from build123d import *

# Parameters (mm, degrees)
SKETCH1_W           = 45
SKETCH1_H           = 45
SKETCH1_R           = 2.6
BOSS_EXTRUDE1_DEPTH = 7.5
SKETCH2_R           = 8.1
CUT_EXTRUDE1_DEPTH  = 6
CUT_EXTRUDE4_START  = -6
SKETCH5_R           = 8.1
CUT_EXTRUDE4_DEPTH  = 6
SKETCH7_W           = 37
SKETCH7_H           = 7
BOSS_EXTRUDE2_DEPTH = 10
CUT_EXTRUDE6_START  = 2
CUT_EXTRUDE6_DEPTH  = 3.6
CUT_EXTRUDE7_START  = -2
SKETCH8_R           = 2.1
CUT_EXTRUDE7_DEPTH  = 41.278836313
SKETCH9_W           = 3
SKETCH9_H           = 7
BOSS_EXTRUDE3_DEPTH = 10
SKETCH10_W          = 7
SKETCH10_H          = 7
BOSS_EXTRUDE4_DEPTH = 2
CHAMFER2_SIZE2      = 7
CHAMFER2_SIZE       = 2
CHAMFER3_SIZE2      = 7
CHAMFER3_SIZE       = 2


with BuildPart() as part:
    # Sketch1 → Boss-Extrude1 (new, symmetric)
    with BuildSketch(Plane.XY):
        Rectangle(SKETCH1_W, SKETCH1_H)
        Circle(SKETCH1_R, mode=Mode.SUBTRACT)
    extrude(amount=BOSS_EXTRUDE1_DEPTH, both=True)

    # Sketch2 → Cut-Extrude1 (cut)
    with BuildSketch(Plane.XY.offset(7.5)):
        Circle(SKETCH2_R)
    extrude(amount=-CUT_EXTRUDE1_DEPTH, mode=Mode.SUBTRACT)

    # Sketch5 → Cut-Extrude4 (cut)
    with BuildSketch(Plane(origin=(0, 0, -7.5), x_dir=(-1, 0, 0), z_dir=(0, 0, -1)).offset(CUT_EXTRUDE4_START)):
        with Locations(Location((0, 0, 0), (0, 0, 180))):
            Circle(SKETCH5_R)
    extrude(amount=CUT_EXTRUDE4_DEPTH, mode=Mode.SUBTRACT)

    # Sketch7 → Boss-Extrude2 (add)
    with BuildSketch(Plane.XZ.offset(22.5)):
        Rectangle(SKETCH7_W, SKETCH7_H)
    extrude(amount=BOSS_EXTRUDE2_DEPTH)

    # Sketch6 → Cut-Extrude6 (cut)
    with BuildSketch(Plane.XY.offset(-7.5).offset(CUT_EXTRUDE6_START)):
        Polygon((19.2, 17.636195996), (15.5, 19.772391992), (11.8, 17.636195996), (11.8, 13.363804004), (15.5, 11.227608008), (19.2, 13.363804004), align=None)
        Polygon((-11.8, 17.636195996), (-15.5, 19.772391992), (-19.2, 17.636195996), (-19.2, 13.363804004), (-15.5, 11.227608008), (-11.8, 13.363804004), align=None)
        Polygon((19.2, -13.363804004), (15.5, -11.227608008), (11.8, -13.363804004), (11.8, -17.636195996), (15.5, -19.772391992), (19.2, -17.636195996), align=None)
        Polygon((-11.8, -13.363804004), (-15.5, -11.227608008), (-19.2, -13.363804004), (-19.2, -17.636195996), (-15.5, -19.772391992), (-11.8, -17.636195996), align=None)
    extrude(amount=CUT_EXTRUDE6_DEPTH, mode=Mode.SUBTRACT)

    # Sketch8 → Cut-Extrude7 (cut, through all)
    with BuildSketch(Plane(origin=(0, 0, -7.5), x_dir=(-1, 0, 0), z_dir=(0, 0, -1)).offset(CUT_EXTRUDE7_START)):
        with Locations((-15.5, 15.5)):
            Circle(SKETCH8_R)
        with Locations((15.5, 15.5)):
            Circle(SKETCH8_R)
        with Locations((15.5, -15.5)):
            Circle(SKETCH8_R)
        with Locations((-15.5, -15.5)):
            Circle(SKETCH8_R)
    extrude(amount=-CUT_EXTRUDE7_DEPTH, mode=Mode.SUBTRACT)

    # Sketch9 → Boss-Extrude3 (add)
    with BuildSketch(Plane.XZ.offset(32.5)):
        with Locations((-17, 0)):
            Rectangle(SKETCH9_W, SKETCH9_H)
        with Locations((17, 0)):
            Rectangle(SKETCH9_W, SKETCH9_H)
    extrude(amount=BOSS_EXTRUDE3_DEPTH)

    # Sketch10 → Boss-Extrude4 (add)
    with BuildSketch(Plane.ZY.offset(18.5)):
        with Locations((0, -39)):
            Rectangle(SKETCH10_W, SKETCH10_H)
    boss_extrude4 = extrude(amount=BOSS_EXTRUDE4_DEPTH)

    # Mirror1: Boss-Extrude4 across plane
    add(boss_extrude4.mirror(Plane(origin=(0, 0, 0), x_dir=(0, 0, 1), z_dir=(1, 0, 0))))

    # Chamfer2
    chamfer2_edges = [part.edges().sort_by_distance(p)[0] for p in [
        (-20.5, -42.5, 0),
    ]]
    chamfer2_side = [part.faces().sort_by_distance(p)[0] for p in [
        (-20.46, -42.5, 0),
    ]]
    chamfer(chamfer2_edges, length=CHAMFER2_SIZE - 0.0001, length2=CHAMFER2_SIZE2 - 0.0001, reference=chamfer2_side[0])  # a hair under: the kernel refuses the full size

    # Chamfer3
    chamfer3_edges = [part.edges().sort_by_distance(p)[0] for p in [
        (20.5, -42.5, 0),
    ]]
    chamfer3_side = [part.faces().sort_by_distance(p)[0] for p in [
        (20.46, -42.5, 0),
    ]]
    chamfer(chamfer3_edges, length=CHAMFER3_SIZE - 0.0001, length2=CHAMFER3_SIZE2 - 0.0001, reference=chamfer3_side[0])  # a hair under: the kernel refuses the full size


solid = part.part
Verification items for the finished model (mm, model axes). A direction names the side the tool comes from. Round coordinates to 2 decimals unless told otherwise and drop trailing zeros. Loops run counter-clockwise (first coordinate to the right, second up) from the corner with the lowest first, then second, coordinate; pieces in that order, holes last. Notation, with made-up numbers: (25, -34) - (31, -34) arc R29 ccw to (31, -13) - close; hole circle Ø7 at (66.5, 80.25). An arc over 180 degrees is marked (long way). Answer in a Markdown table with one row per item. Add a question column.
Q1. Material ranges on line 1 (Y direction, x = 15.5, z = 4.25); line 2 (Y direction, x = 0, z = -4.75); line 3 (Z direction, x = 14, y = 12.5), recorded low to high.
Q2. Release check for a two-part mould opening along Z. For faces 5 (the face through (15.5, -37, 0)), 6 (the face through (11.8, 16, -4)), 7 (the face through (0, 10, 7.5)) record: pulls with the +Z half, pulls with the -Z half, needs draft (parallel to the pull), parting line crosses it, or undercut.
Q3. Section check B-B on x = 0. Enter the section's corners in (y, z).
Q4. Section check D-D on x = -9. Enter the section's corners in (y, z), plus the area to 3 significant figures.
Q5. Section check C-C on y = 15.5. Enter the section's corners in (x, z), plus the area to 3 significant figures.
Q6. Gauge pin test, flat ends, axial feed: pin 1 (3.5 mm diameter, centred on y = -28, z = 0, fed in from -X); pin 2 (1.5 mm diameter, centred on x = 11, z = 0, fed in from -Y); pin 3 (2 mm diameter, centred on x = 5, y = -35, fed in from +Z); pin 4 (3.5 mm diameter, centred on y = -30.5, z = -1.5, fed in from +X). Record the tip position at first contact, or that the pin passes through.
Q7. Section check A-A on z = 4.75. Enter the section's corners in (x, y).
Q8. Tool access check on faces 1 (the face through (-18.5, -29, 0)), 2 (the face through (-1.756, 7.907, -4.458)), 3 (the face through (19.2, 15, -4)), 4 (the face through (-15.5, -37, 0)). Record the directions out of +Z, -Z, +X, -X, +Y, -Y that give a thin tool (end or side, any length) a straight path to the whole face; none if there is none.
Found:
| question | item | result |
|---|---|---|
| 1 | line 1 | y = -22.5 to -17.6, -13.4 to 13.4, 17.6 to 22.5 |
| 1 | line 2 | y = -22.5 to -8.1, 8.1 to 22.5 |
| 1 | line 3 | z = -7.5 to -5.5, -1.9 to 7.5 |
| 2 | face 5 | needs draft |
| 2 | face 6 | undercut |
| 2 | face 7 | pulls with the +Z half |
| 3 | outline | (-32.5, -3.5) - (-22.5, -3.5) - (-22.5, -7.5) - (-8.1, -7.5) - (-8.1, -1.5) - (-2.6, -1.5) - (-2.6, 1.5) - (-8.1, 1.5) - (-8.1, 7.5) - (-22.5, 7.5) - (-22.5, 3.5) - (-32.5, 3.5) - close; (2.6, -1.5) - (8.1, -1.5) - (8.1, -7.5) - (22.5, -7.5) - (22.5, 7.5) - (8.1, 7.5) - (8.1, 1.5) - (2.6, 1.5) - close |
| 4 | outline | (-32.5, -3.5) - (-22.5, -3.5) - (-22.5, -7.5) - (22.5, -7.5) - (22.5, 7.5) - (-22.5, 7.5) - (-22.5, 3.5) - (-32.5, 3.5) - close |
| 4 | area | 745 mm² |
| 5 | outline | (-22.5, -7.5) - (22.5, -7.5) - (22.5, 7.5) - (17.6, 7.5) - (17.6, -1.9) - (19.2, -1.9) - (19.2, -5.5) - (11.8, -5.5) - (11.8, -1.9) - (13.4, -1.9) - (13.4, 7.5) - (-13.4, 7.5) - (-13.4, -1.9) - (-11.8, -1.9) - (-11.8, -5.5) - (-19.2, -5.5) - (-19.2, -1.9) - (-17.6, -1.9) - (-17.6, 7.5) - (-22.5, 7.5) - close |
| 5 | area | 543 mm² |
| 6 | pin 1 | stops at x = -18.5 |
| 6 | pin 2 | stops at y = -32.5 |
| 6 | pin 3 | passes through |
| 6 | pin 4 | stops at x = 18.5 |
| 7 | outline | (-22.5, -22.5) - (22.5, -22.5) - (22.5, 22.5) - (-22.5, 22.5) - close; hole circle Ø4.2 at (-15.5, -15.5); hole circle Ø4.2 at (-15.5, 15.5); hole circle Ø16.2 at (0, 0); hole circle Ø4.2 at (15.5, -15.5); hole circle Ø4.2 at (15.5, 15.5) |
| 8 | face 1 | +Z, -Z, -X |
| 8 | face 2 | -Z |
| 8 | face 3 | none |
| 8 | face 4 | +Z, -Z, -Y |
